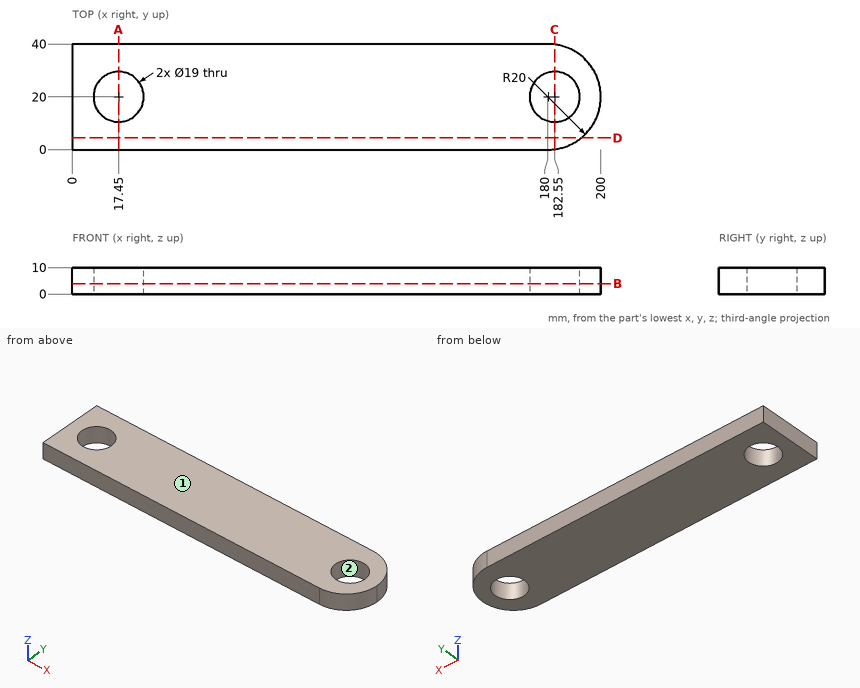
Drawing for the job (mm, zero at the part's lowest x, y, z). Give positions to 0.01 mm unless a question says otherwise; leave off trailing zeros. Order: outer loops, then holes, each group sorted by start corner. A loop starts at its lowest first (then second) coordinate and runs counter-clockwise, first axis right, second up. Notation, with made-up numbers: M -27.75,28 L 3.25,28 A11 cw 3.25,33 Z; hole C 76,51.25 d7. An arc over 180 degrees is marked long. Write item = value, one per line. Start each with the question number.
(1) Two-plate mould, pull along X, no slides. Class the marked faces 1 and 2: released by +X, released by -X, zero draft, split by the parting line, or undercut.
(2) Slice it at D-D on y = 4.5. Write the cut outline in (x, z), plus the area to 3 significant figures.
(3) Slice it at A-A on x = 17.45. Write the cut outline in (y, z).
(4) Slice it at B-B on z = 4. Write the cut outline in (x, y).
(5) Probe L1, parallel to Y at x = 17.45, z = 5.25; L2, parallel to X at y = 26, z = 2.75; L3, parallel to X at y = 22, z = 9.75. List the from-to ranges inside material, lowest first. Write a range as [from, to].
(6) Pin check, flat tip, straight feed: pin 1 Ø5 at (y, z) = (7, 1) entering from +X. Stop position of the tip, or through.
(7) Slice it at C-C on x = 182.55. Write the cut outline in (y, z).
Responses:
q1.face_1 = zero draft
q1.face_2 = undercut
q2.outline = M 0,0 L 192.64,0 L 192.64,10 L 0,10 Z
q2.area = 1,930 mm2
q3.outline = M 0,0 L 10.5,0 L 10.5,10 L 0,10 Z; M 29.5,0 L 40,0 L 40,10 L 29.5,10 Z
q4.outline = M 0,0 L 180,0 A20 ccw 200,20 A20 ccw 180,40 L 0,40 Z; hole C 17.45,20 d19; hole C 182.55,20 d19
q5.L1 = [0, 10.5], [29.5, 40]
q5.L2 = [0, 10.08], [24.82, 175.18], [189.92, 199.08]
q5.L3 = [0, 8.16], [26.74, 173.26], [191.84, 199.9]
q6.pin_1 = 197.02
q7.outline = M 0.16,0 L 10.5,0 L 10.5,10 L 0.16,10 Z; M 29.5,0 L 39.84,0 L 39.84,10 L 29.5,10 Z
